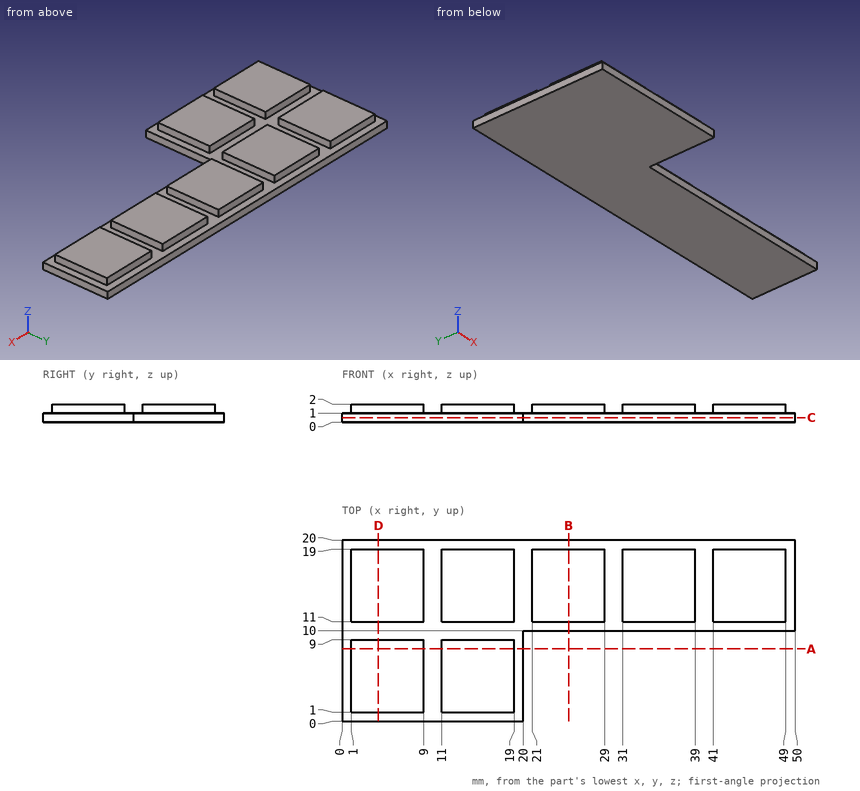
Drawing for the job (mm, zero at the part's lowest x, y, z). Round coordinates to 2 decimals unless told otherwise and drop trailing zeros. Write each loop counter-clockwise with the first axis right and the second up, starting at its lowest first coordinate (ties: lowest second). Pieces come first, ordered by that corner, then holes.
Item 1: Band-saw the part on B-B on x = 25. Write the cut outline in (y, z).
Filled in:
outline: (10, 0) - (20, 0) - (20, 1) - (19, 1) - (19, 2) - (11, 2) - (11, 1) - (10, 1) - close
Item 2: Drill centre lines: L1, parallel to X at y = 12.75, z = 1.4; L2, parallel to X at y = 3.25, z = 1.4. Where is each one in solid material? Low to high.
Filled in:
L1: x = 1 to 9, 11 to 19, 21 to 29, 31 to 39, 41 to 49
L2: x = 1 to 9, 11 to 19
Item 3: Band-saw the part on C-C on z = 0.5. Write the cut outline in (x, y), then the cut area to 3 significant figures.
Filled in:
outline: (0, 0) - (20, 0) - (20, 10) - (50, 10) - (50, 20) - (0, 20) - close
area: 700 mm2
Item 4: Drop flat-ended pins along their axis: pin 1 Ø8 at (x, y) = (26.5, 14) entering from -Z; pin 2 Ø0.8 at (y, z) = (13, 1.5) entering from -X; pin 3 Ø0.8 at (x, z) = (5.5, 1.5) entering from -Y; pin 4 Ø0.8 at (x, z) = (32.5, 0.5) entering from -Y. Give the stop position or say it passes through.
Filled in:
pin 1: stops at z = 0
pin 2: stops at x = 1
pin 3: stops at y = 1
pin 4: stops at y = 10
Item 5: Band-saw the part on A-A on y = 8. Write the cut outline in (x, z), then the cut area to 3 significant figures.
Filled in:
outline: (0, 0) - (20, 0) - (20, 1) - (19, 1) - (19, 2) - (11, 2) - (11, 1) - (9, 1) - (9, 2) - (1, 2) - (1, 1) - (0, 1) - close
area: 36.0 mm2
